Part model, mm, in its own coordinate system. Round coordinates to 2 decimals unless told otherwise and drop trailing zeros. Order: outer loops, then holes, each group sorted by start corner. A loop starts at its lowest first (then second) coordinate and runs counter-clockwise, first axis right, second up. Notation, with made-up numbers: (75, 27.5) - (81, 27.5) arc R30 ccw to (81, 60.5) - close; hole circle Ø4 at (18, 21.5). An arc over 180 degrees is marked (long way). Answer as a JSON object with one key per item and string values.
```python
from build123d import *

# Parameters (mm, degrees)
SKETCH1_R           = 1.55575
BOSS_EXTRUDE1_DEPTH = 1.524
FILLET1_R           = 5.08
FILLET2_R           = 45.72
FILLET3_R           = 8.89


with BuildPart() as part:
    # Sketch1 → Boss-Extrude1 (new body)
    with BuildSketch(Plane.XY):
        Polygon((0, 49.0982), (0, 76.2), (15.24, 76.2), (15.24, 0), (0, 0), (0, 27.1018), (-109.22, 27.1018), (-109.22, 49.0982), align=None)
        with Locations(Location((7.4041, 68.7959, 0), (0, 0, 180))):
            Circle(SKETCH1_R, mode=Mode.SUBTRACT)
        with Locations(Location((7.4041, 7.4041, 0), (0, 0, 180))):
            Circle(SKETCH1_R, mode=Mode.SUBTRACT)
    extrude(amount=BOSS_EXTRUDE1_DEPTH)

    # Fillet1
    fillet1_edges = [part.edges().sort_by_distance(p)[0] for p in [
        (-109.22, 27.1018, 0.762),
        (-109.22, 49.0982, 0.762),
    ]]
    fillet(fillet1_edges, radius=FILLET1_R)

    # Fillet2
    # the kernel refuses this fillet: 45.72 mm, written as the material it adds along each edge
    with BuildSketch(Plane(origin=(0, 27.1018, 0), x_dir=(-1, 0, 0), z_dir=(0, 0, 1))) as fillet2_piece_1:
        with BuildLine():
            CenterArc((41.757406873, 45.72), FILLET2_R, 204.030458178, 65.969541822)
            Line((0, 27.1018), (-0.835148137, 26.729436))
            ThreePointArc((-0.835148137, 26.729436), (-0.9144, 13.5509), (-0.9144, 0))
            Line((-0.9144, 0), (0, -0.9144))
            Line((0, -0.9144), (41.757406873, -0.9144))
            Line((41.757406873, -0.9144), (41.757406873, 0))
        make_face()
    extrude(amount=1.524)
    with BuildSketch(Plane(origin=(0, 49.0982, 0), x_dir=(-1, 0, 0), z_dir=(0, 0, 1))) as fillet2_piece_2:
        with BuildLine():
            CenterArc((41.757406873, -45.72), FILLET2_R, 90, 65.969541822)
            Line((0, -27.1018), (-0.835148137, -26.729436))
            ThreePointArc((-0.835148137, -26.729436), (-0.9144, -13.5509), (-0.9144, 0))
            Line((-0.9144, 0), (0, 0.9144))
            Line((0, 0.9144), (41.757406873, 0.9144))
            Line((41.757406873, 0.9144), (41.757406873, 0))
        make_face()
    extrude(amount=1.524)

    # Fillet3
    fillet3_edges = [part.edges().sort_by_distance(p)[0] for p in [
        (0, 76.2, 0.762),
        (0, 0, 0.762),
    ]]
    fillet(fillet3_edges, radius=FILLET3_R)


solid = part.part
```
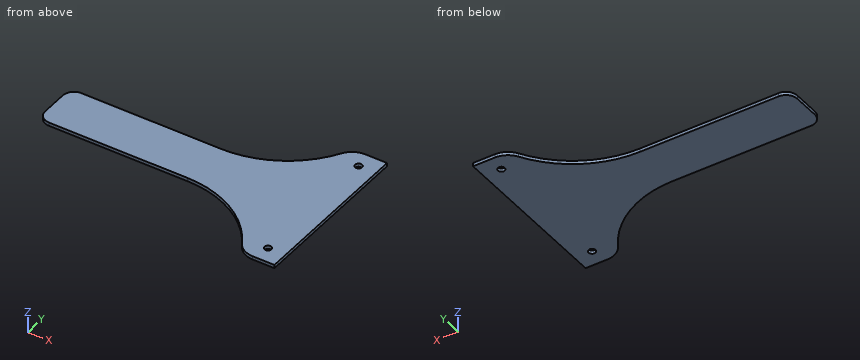
Item 1: Cut at C-C (y = 66). Write the cut outline in (x, z), plus the area to 3 significant figures.
Taken from the geometry:
{"outline": "(-6.26, 0) - (15.24, 0) - (15.24, 1.52) - (-6.26, 1.52) - close", "area": "32.8 mm2"}
Item 2: Cut at A-A (z = 0.9). Write the cut outline in (x, y).
Taken from the geometry:
{"outline": "(-109.22, 32.18) arc R5.08 ccw to (-104.14, 27.1) - (-41.76, 27.1) arc R45.72 cw to (-2.26, 4.41) arc R8.89 ccw to (5.42, 0) - (15.24, 0) - (15.24, 76.2) - (5.42, 76.2) arc R8.89 ccw to (-2.26, 71.79) arc R45.72 cw to (-41.76, 49.1) - (-104.14, 49.1) arc R5.08 ccw to (-109.22, 44.02) - close; hole circle Ø3.11 at (7.4, 7.4); hole circle Ø3.11 at (7.4, 68.8)"}
Item 3: Probe L1, parallel to Y at x = 7, z = 0.6; L2, parallel to Y at x = -85, z = 0.25; L3, parallel to Y at x = -19, z = 1.1. List the from-to ranges inside material, lowest first. Write a range as from..to.
Taken from the geometry:
{"L1": "0..5.9, 8.91..67.29, 70.3..76.2", "L2": "27.1..49.1", "L3": "21.04..55.16"}
Item 4: Drop flat-ended pins along their axis: P1, Ø0.8, axis at x = -86, z = 0.5, coming from the -Y side; P2, Ø1.9, axis at x = 7.4, y = 7.4, coming from the +Z side. Give the stop position or say it passes through.
Taken from the geometry:
{"P1": "y = 27.1", "P2": "through"}
Item 5: Cut at B-B (x = -85.5). Write the cut outline in (y, z), plus the area to 3 significant figures.
Taken from the geometry:
{"outline": "(27.1, 0) - (49.1, 0) - (49.1, 1.52) - (27.1, 1.52) - close", "area": "33.5 mm2"}
